The figure shows three views and two pictorial views of one solid part (mm, origin at its lowest corner). Answer the questions. Coordinates: 2 decimals unless noted, no trailing zeros. Order: outer loops, then holes, each group sorted by start corner. A loop starts at its lowest first (then second) coordinate and runs counter-clockwise, first axis right, second up. Notation, with made-up numbers: (79.5, -39) - (112.5, -39) arc R19 ccw to (112.5, -6) - close; hole circle Ø8 at (23, -1.5). An arc over 180 degrees is marked (long way). Use one line per item in the form item = value. Start each with the question number.
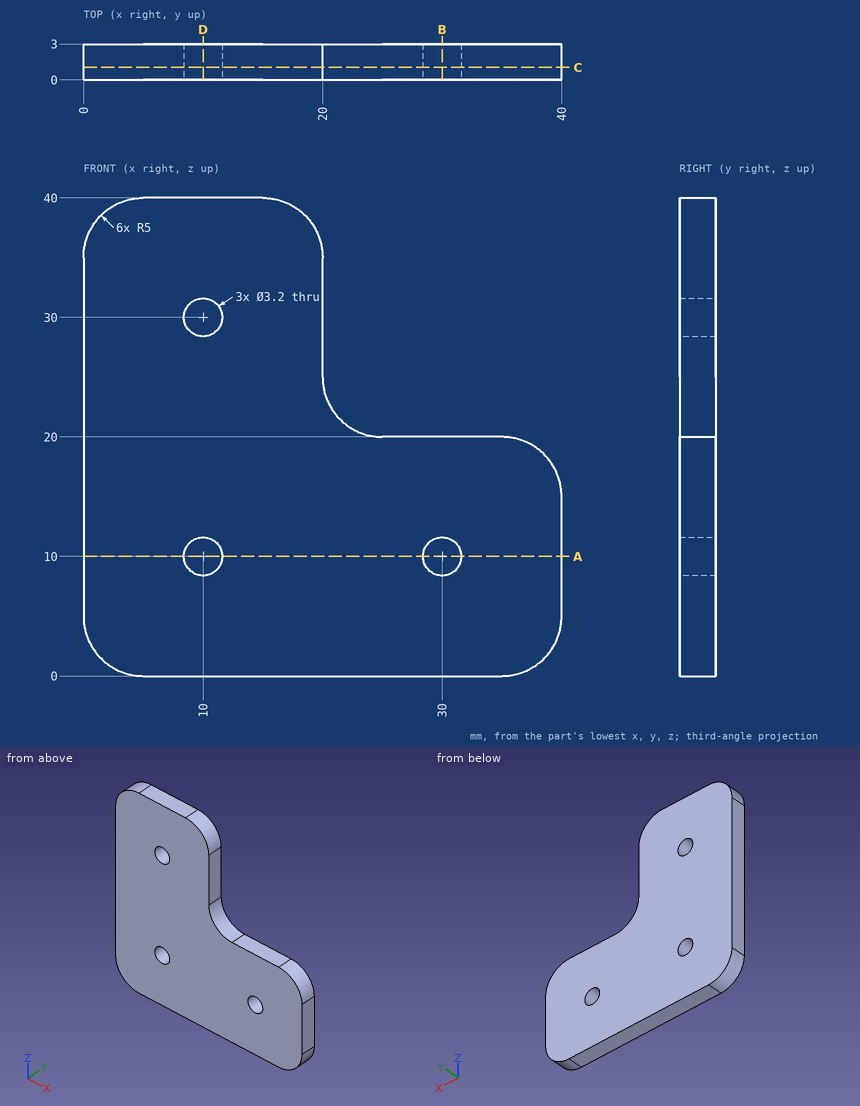
Q1. A cutting plane is placed at B-B (x = 30). Give the vertices of the cut face in (y, z).
Q2. A cutting plane is placed at C-C (y = 1.05). Give the vertices of the cut face in (x, z).
Q3. Consider probe 1 along X at (y, z) = (2.3, 10); probe 2 along X at (y, z) = (1.35, 30); probe 3 along X at (y, z) = (2.2, 25). Determine where each line is inside the solid, lowest interval first.
Q4. A cutting plane is placed at D-D (x = 10). Give the vertices of the cut face in (y, z).
Q5. Given P1, Ø8, axis at x = 16.5, z = 19, coming from the -Y side; P2, Ø1.5, axis at x = 18, y = 2.5, coming from the +Z side, each flat-ended and moving along its own axis, determine where each tip first touches the part or whether it passes through.
Q6. A cutting plane is placed at A-A (z = 10). Give the vertices of the cut face in (x, y).
Result sheet:
q1.outline = (0, 0) - (3, 0) - (3, 8.4) - (0, 8.4) - close; (0, 11.6) - (3, 11.6) - (3, 20) - (0, 20) - close
q2.outline = (0, 5) arc R5 ccw to (5, 0) - (35, 0) arc R5 ccw to (40, 5) - (40, 15) arc R5 ccw to (35, 20) - (25, 20) arc R5 cw to (20, 25) - (20, 35) arc R5 ccw to (15, 40) - (5, 40) arc R5 ccw to (0, 35) - close; hole circle Ø3.2 at (10, 10); hole circle Ø3.2 at (10, 30); hole circle Ø3.2 at (30, 10)
q3.probe_1 = 0 to 8.4, 11.6 to 28.4, 31.6 to 40
q3.probe_2 = 0 to 8.4, 11.6 to 20
q3.probe_3 = 0 to 20
q4.outline = (0, 0) - (3, 0) - (3, 8.4) - (0, 8.4) - close; (0, 11.6) - (3, 11.6) - (3, 28.4) - (0, 28.4) - close; (0, 31.6) - (3, 31.6) - (3, 40) - (0, 40) - close
q5.P1 = 0
q5.P2 = 39.47
q6.outline = (0, 0) - (8.4, 0) - (8.4, 3) - (0, 3) - close; (11.6, 0) - (28.4, 0) - (28.4, 3) - (11.6, 3) - close; (31.6, 0) - (40, 0) - (40, 3) - (31.6, 3) - close
